Study the drawing (mm; zero at the part's minimum x, y, z) and answer. A direction names the side the tool comes from. Coordinates: 2 decimals unless noted, no trailing zeros. Order: outer loops, then holes, each group sorted by start corner. A loop starts at its lowest first (then second) coordinate and runs counter-clockwise, first axis right, second up.
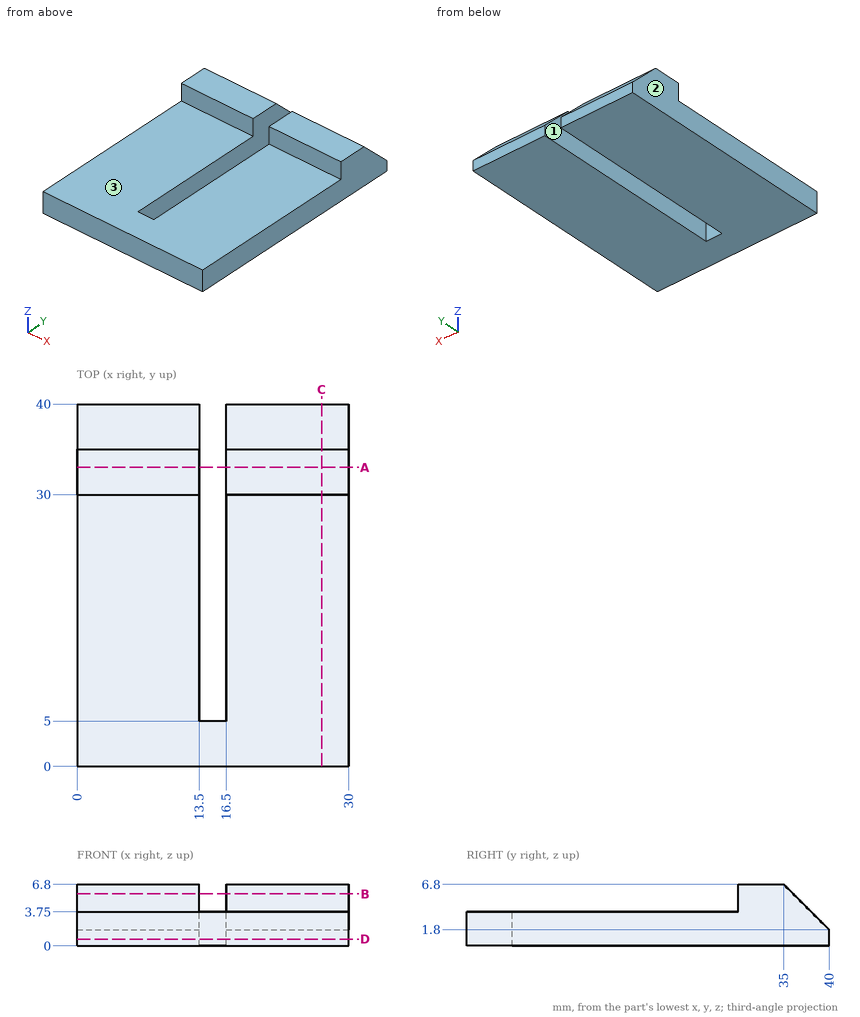
(1) Find section A-A (y = 33). Write down the section's boundary in (x, z), and give its area (3 significant figures).
(2) Each of these flat-tipped pins is pushed along its axis until it touches: pin 1 Ø1.5 at (x, z) = (25, 6) entering from -Y; pin 2 Ø3 at (x, z) = (14, 3.5) entering from +Y; pin 3 Ø3 at (x, z) = (9, 4) entering from +Y. Where does it stop, or does it pass through?
(3) Find section C-C (x = 27). Write down the section's boundary in (y, z), and give its area (3 significant figures).
(4) Consider line 1 (X direction, y = 16, z = 2.5); line 2 (Z direction, x = 5.75, y = 22); line 3 (Z direction, x = 12.5, y = 36). Determine where each line is inside the solid, lowest interval first.
(5) For the marked faces 1, 2 and 3, determine the directions among +Z, -Z, +X, -X, +Y, -Y from which every point of the face is accessible in a straight line to the end or side of a thin tool.
(6) Find section D-D (z = 0.75). Write down the section's boundary in (x, y).
(7) Find section B-B (z = 5.75). Write down the section's boundary in (x, y).
Findings below:
1. outline: (0, 0) - (13.5, 0) - (13.5, 6.8) - (0, 6.8) - close; (16.5, 0) - (30, 0) - (30, 6.8) - (16.5, 6.8) - close
1. area: 184 mm2
2. pin 1: stops at y = 30
2. pin 2: stops at y = 39.71
2. pin 3: stops at y = 39.3
3. outline: (0, 0) - (40, 0) - (40, 1.8) - (35, 6.8) - (30, 6.8) - (30, 3.75) - (0, 3.75) - close
3. area: 168 mm2
4. line 1: x = 0 to 13.5, 16.5 to 30
4. line 2: z = 0 to 3.75
4. line 3: z = 0 to 5.8
5. face 1: +Z, -Z, +Y
5. face 2: +Z, -Z, -X, +Y, -Y
5. face 3: +Z, +X, -X, -Y
6. outline: (0, 0) - (30, 0) - (30, 40) - (16.5, 40) - (16.5, 5) - (13.5, 5) - (13.5, 40) - (0, 40) - close
7. outline: (0, 30) - (13.5, 30) - (13.5, 36.05) - (0, 36.05) - close; (16.5, 30) - (30, 30) - (30, 36.05) - (16.5, 36.05) - close
